from build123d import *

# Parameters (mm, degrees)
F0_R     = 1.27
F1_DEPTH = 25.4
F2_DEPTH = 2.54
F4_DEPTH = 2.54
F8_DEPTH = 20.32


# Not quite as in the source:
# - a feature names something its author has since deleted; it is built from what else it names


with BuildPart() as f1:
    # F0 (on Right) → F1 (new body)
    with BuildSketch(Plane.YZ):
        with BuildLine():
            Line((-50.8, 0), (-9.8610056184, 0))
            Line((-9.8610056184, 0), (-0.6510920475, -8.592966345))
            ThreePointArc((-0.6510920475, -8.592966345), (2.514052834, -9.3825729095), (4.8603454258, -7.1161811248))
            Line((4.8603454258, -7.1161811248), (8.5398813724, 4.9305028092))
            Line((8.5398813724, 4.9305028092), (43.9940905122, 25.4))
            Line((43.9940905122, 25.4), (40.2770972977, 26.1869323345))
            Line((40.2770972977, 26.1869323345), (8.3697336352, 7.7652073348))
            ThreePointArc((8.3697336352, 7.7652073348), (7.4060334479, 7.6383337982), (6.6348813724, 8.2300595976))
            Line((6.6348813724, 8.2300595976), (-9.8610056184, 36.8017739816))
            Line((-9.8610056184, 36.8017739816), (-9.8610056184, 3.81))
            ThreePointArc((-9.8610056184, 3.81), (-10.2329800063, 2.9119743879), (-11.1310056184, 2.54))
            Line((-11.1310056184, 2.54), (-47.9744556178, 2.54))
            Line((-47.9744556178, 2.54), (-50.8, 0))
        make_face()
        with Locations((1.6435009364, -6.1336289969)):
            Circle(F0_R, mode=Mode.SUBTRACT)
        with BuildLine():
            Line((-1.0208864232, 2.54), (-6.0510056184, 2.54))
            ThreePointArc((-6.0510056184, 2.54), (-6.9490312305, 2.9119743879), (-7.3210056184, 3.81))
            Line((-7.3210056184, 3.81), (-7.3210056184, 22.5826604048))
            ThreePointArc((-7.3210056184, 22.5826604048), (-6.3797058057, 23.8093862042), (-4.9511533556, 23.2176604048))
            Line((-4.9511533556, 23.2176604048), (4.4351768468, 6.9600595976))
            ThreePointArc((4.4351768468, 6.9600595976), (4.5620503834, 5.9963594103), (3.970324584, 5.2252073348))
            Line((3.970324584, 5.2252073348), (-0.3858864232, 2.7101477372))
            ThreePointArc((-0.3858864232, 2.7101477372), (-0.6921862359, 2.5832742006), (-1.0208864232, 2.54))
        make_face(mode=Mode.SUBTRACT)
    extrude(amount=F1_DEPTH)

    # F0 (on Right) → F2 (join)
    with BuildSketch(Plane.YZ):
        with BuildLine():
            Line((-9.8610056184, 36.8017739816), (-47.9744556178, 2.54))
            Line((-47.9744556178, 2.54), (-11.1310056184, 2.54))
            ThreePointArc((-11.1310056184, 2.54), (-10.2329800063, 2.9119743879), (-9.8610056184, 3.81))
            Line((-9.8610056184, 3.81), (-9.8610056184, 36.8017739816))
        make_face()
        with BuildLine():
            Line((-8.3631146249, 36.484652376), (-9.8610056184, 36.8017739816))
            Line((-9.8610056184, 36.8017739816), (6.6348813724, 8.2300595976))
            ThreePointArc((6.6348813724, 8.2300595976), (7.4060334479, 7.6383337982), (8.3697336352, 7.7652073348))
            Line((8.3697336352, 7.7652073348), (40.2770972977, 26.1869323345))
            Line((40.2770972977, 26.1869323345), (-8.3631146249, 36.484652376))
        make_face()
    extrude(amount=F2_DEPTH)

    # F3 (on face) → F4 (join)
    with BuildSketch(Plane.YZ.offset(25.4)):
        with BuildLine():
            Line((-9.8610056184, 3.81), (-9.8610056184, 36.8017739816))
            Line((-9.8610056184, 36.8017739816), (-47.9744556178, 2.54))
            Line((-47.9744556178, 2.54), (-11.1310056184, 2.54))
            ThreePointArc((-11.1310056184, 2.54), (-10.2329800063, 2.9119743879), (-9.8610056184, 3.81))
        make_face()
        with BuildLine():
            Line((40.2770972977, 26.1869323345), (-9.8610056184, 36.8017739816))
            Line((-9.8610056184, 36.8017739816), (6.6348813724, 8.2300595976))
            ThreePointArc((6.6348813724, 8.2300595976), (7.4060334479, 7.6383337982), (8.3697336352, 7.7652073348))
            Line((8.3697336352, 7.7652073348), (40.2770972977, 26.1869323345))
        make_face()
    extrude(amount=-F4_DEPTH)

    # F7 (on offset) → F8 (cut)
    with BuildSketch(Plane.YZ.offset(2.54)):
        with BuildLine():
            Line((8.5398813724, 4.9305028092), (0.2947045256, 0.1701477372))
            ThreePointArc((0.2947045256, 0.1701477372), (-0.0115952871, 0.0432742006), (-0.3402954744, 0))
            Line((-0.3402954744, 0), (-9.8610056184, 0))
            Line((-9.8610056184, 0), (-0.6510920475, -8.592966345))
            ThreePointArc((-0.6510920475, -8.592966345), (2.514052834, -9.3825729095), (4.8603454258, -7.1161811248))
            Line((4.8603454258, -7.1161811248), (8.5398813724, 4.9305028092))
        make_face()
    extrude(amount=F8_DEPTH, mode=Mode.SUBTRACT)


solid = f1.part
Part model, mm, in its own coordinate system. A direction names the side the tool comes from. Coordinates: 2 decimals unless noted, no trailing zeros. Order: outer loops, then holes, each group sorted by start corner. A loop starts at its lowest first (then second) coordinate and runs counter-clockwise, first axis right, second up. Notation, with made-up numbers: M -2.5,-35 L 9.5,-35 A18 cw 9.5,-21 Z; hole C 47,-34 d8. An arc over 180 degrees is marked long. Use a Markdown table: item, result.
(1) Cut at B-B on y = 1.5. Write the cut outline in (x, z), then the cut area to 3 significant figures.
A:
| item | result |
|---|---|
| outline | M 0,-9.49 L 2.54,-9.49 L 2.54,-7.4 L 0,-7.4 Z; M 0,-4.87 L 2.54,-4.87 L 2.54,0.87 L 22.86,0.87 L 22.86,-4.87 L 25.4,-4.87 L 25.4,3.8 L 0,3.8 Z; M 0,12.04 L 25.4,12.04 L 25.4,34.4 L 22.86,34.4 L 22.86,17.12 L 2.54,17.12 L 2.54,34.4 L 0,34.4 Z; M 22.86,-9.49 L 25.4,-9.49 L 25.4,-7.4 L 22.86,-7.4 Z |
| area | 331 mm^2 |
(2) Cut at A-A on z = 11.5. Write the cut outline in (x, y).
A:
| item | result |
|---|---|
| outline | M 0,-38.01 L 2.54,-38.01 L 2.54,-9.86 L 22.86,-9.86 L 22.86,-38.01 L 25.4,-38.01 L 25.4,-7.32 L 0,-7.32 Z; M 0,1.81 L 25.4,1.81 L 25.4,19.92 L 0,19.92 Z; hole M 2.54,4.75 L 22.86,4.75 L 22.86,14.84 L 2.54,14.84 Z |
(3) Tool access for faces 4 (the flat face through (13, -29, 2.54)), 5 (the flat face through (12.52, -0.32, 15.2)), 6 (the flat face through (13, -26, 0)): list every direction of +Z, -Z, +X, -X, +Y, -Y with a clear straight run to the whole face (end or side of a thin tool).
A:
| item | result |
|---|---|
| face 4 | +Z, -Y |
| face 5 | +X, -X |
| face 6 | -Z, -Y |
(4) Pull direction X, two halves, no side cores. Call faces 1 (the flat face through (22.86, -21, 12)), 2 (the flat face through (25.4, -4, 24)), 3 (the flat face through (13, -7.321, 13)): released by +X, released by -X, zero draft, split by the parting line, or undercut.
A:
| item | result |
|---|---|
| face 1 | undercut |
| face 2 | released by +X |
| face 3 | zero draft |
(5) Cut at D-D on z = -1. Write the cut outline in (x, y).
A:
| item | result |
|---|---|
| outline | M 0,-8.79 L 2.54,-8.79 L 2.54,6.73 L 0,6.73 Z; M 22.86,-8.79 L 25.4,-8.79 L 25.4,6.73 L 22.86,6.73 Z |
(6) Probe L1, parallel to Y at x = 11.25, z = 12; L2, parallel to X at y = 3.5, z = 20; L3, parallel to Y at x = 8.5, z = 12.5. List the from-to ranges inside material, lowest first.
A:
| item | result |
|---|---|
| L1 | y = -9.86 to -7.32, 1.53 to 4.46, 15.7 to 20.78 |
| L2 | x = 0 to 2.54, 22.86 to 25.4 |
| L3 | y = -9.86 to -7.32, 1.24 to 4.17, 16.57 to 21.65 |
(7) Flat gauge pins, fed straight in: pin 1 (8 mm diameter, centred on x = 7, y = -19.5, fed in from -Z); pin 2 (6 mm diameter, centred on x = 17, z = 32, fed in from +Y); pin 3 (1 mm diameter, centred on x = 5.5, y = 10.5, fed in from -Z). Where does each tip first touch, or does it go through?
A:
| item | result |
|---|---|
| pin 1 | stops at z = 0 |
| pin 2 | stops at y = -5.36 |
| pin 3 | stops at z = 5.77 |
(8) Cut at C-C on x = 10.5. Write the cut outline in (y, z), then the cut area to 3 significant figures.
A:
| item | result |
|---|---|
| outline | M -50.8,0 L -0.34,0 A1.27 ccw 0.29,0.17 L 43.99,25.4 L 40.28,26.19 L 8.37,7.77 A1.27 cw 6.63,8.23 L -9.86,36.8 L -9.86,3.81 A1.27 cw -11.13,2.54 L -47.97,2.54 Z; hole M -7.32,3.81 A1.27 ccw -6.05,2.54 L -1.02,2.54 A1.27 ccw -0.39,2.71 L 3.97,5.23 A1.27 ccw 4.44,6.96 L -4.95,23.22 A1.27 ccw -7.32,22.58 Z |
| area | 404 mm^2 |
